Geometry: final body of the model. Coordinates: model frame, mm. A direction names the side the tool comes from. Round coordinates to 2 decimals unless told otherwise and drop trailing zeros. Write each loop counter-clockwise with the first axis right and the second up, starting at its lowest first coordinate (ties: lowest second). Pieces come first, ordered by that corner, then holes. Notation, with made-up numbers: (72.25, 14.25) -> (78.25, 14.25) arc R14 cw to (78.25, 29.25) -> close; hole circle Ø1 at (-10, 67.5). An arc over 180 degrees is marked (long way). Use one line per item in the form item = value. Start each with the question number.
1. Reachability of faces 1 (the face through (1.5, 0.07, -2.54)), 2 (the face through (0, 0, 5)), 3 (the face through (1.8, 0, 5)) from +Z, -Z, +X, -X, +Y, -Y: full face, straight path, thin tool, end or side. Return the list, or none.
2. Cut plane D-D, the plane y = 1.65. Return the cut outline in (x, z).
3. Draft query along Y for faces 4 (the face through (-1.5, 0.07, 7.46)), 5 (the face through (0.913, 1.552, 4.93)), 6 (the face through (-0.913, -1.552, 4.93)). Return one class per face: pulls with the +Y half, pulls with the -Y half, needs draft (parallel to the pull), parting line crosses it, or undercut.
4. Pin query (flat end, axial travel): pin 1 Ø1.5 at (x, y) = (-0.5, 0.5) entering from +Z; pin 2 Ø2 at (x, z) = (0.5, 2.5) entering from -Y. Return the tip coordinate at first contact, or that it passes through.
5. Cut plane A-A, the plane z = 2.5. Return the cut outline in (x, y), plus the area to 3 significant figures.
6. Cut plane B-B, the plane x = 1.05. Return the cut outline in (y, z).
7. Line query: L1, parallel to X at y = 0, z = 8.15; L2, parallel to Z at x = 1.2, y = -0.15; L3, parallel to Z at x = -1, y = -1.2. Output: solid intervals per line, ascending.
8. Cut plane C-C, the plane y = 0.25. Return the cut outline in (x, z).
```python
from build123d import *

# Parameters (mm, degrees)
SKETCH_1_R      = 1.5
EXTRUDE_1_DEPTH = 10
SKETCH_2_R      = 1.5
EXTRUDE_2_DEPTH = 5


with BuildPart() as part:
    # 草图1 → 凸台-拉伸1 (new body)
    with BuildSketch(Plane.XY):
        Polygon((0, 2.078460969), (-1.8, 1.039230485), (-1.8, -1.039230485), (0, -2.078460969), (1.8, -1.039230485), (1.8, 1.039230485), align=None)
        Circle(SKETCH_1_R, mode=Mode.SUBTRACT)
    extrude(amount=EXTRUDE_1_DEPTH)

    # 草图2 → 凸台-拉伸2 (add, symmetric)
    with BuildSketch(Plane(origin=(0, 0, 0), x_dir=(-1, 0, 0), z_dir=(0, 0, -1))):
        Circle(SKETCH_2_R)
    extrude(amount=EXTRUDE_2_DEPTH, both=True)


solid = part.part
```
Outcome:
q1.face_1 = -Z
q1.face_2 = +Z
q1.face_3 = +Z, -Z, +X, +Y, -Y
q2.outline = (-0.74, 0) -> (0.74, 0) -> (0.74, 10) -> (-0.74, 10) -> close
q3.face_4 = undercut
q3.face_5 = pulls with the +Y half
q3.face_6 = pulls with the -Y half
q4.pin_1 = 5
q4.pin_2 = -2.08
q5.outline = (-1.8, -1.04) -> (0, -2.08) -> (1.8, -1.04) -> (1.8, 1.04) -> (0, 2.08) -> (-1.8, 1.04) -> close
q5.area = 11.2 mm^2
q6.outline = (-1.47, 0) -> (-1.07, 0) -> (-1.07, -5) -> (1.07, -5) -> (1.07, 0) -> (1.47, 0) -> (1.47, 10) -> (1.07, 10) -> (1.07, 5) -> (-1.07, 5) -> (-1.07, 10) -> (-1.47, 10) -> close
q7.L1 = -1.8 to -1.5, 1.5 to 1.8
q7.L2 = -5 to 5
q7.L3 = 0 to 10
q8.outline = (-1.8, 0) -> (-1.48, 0) -> (-1.48, -5) -> (1.48, -5) -> (1.48, 0) -> (1.8, 0) -> (1.8, 10) -> (1.48, 10) -> (1.48, 5) -> (-1.48, 5) -> (-1.48, 10) -> (-1.8, 10) -> close
